```python
from build123d import *

# Parameters (mm, degrees)
F1_DEPTH = 15.748
F2_W     = 38.1
F2_H     = 11.4949838928
F3_DEPTH = 38.1
F4_R     = 19.04999
F6_D     = 15.875
F7_R     = 15.875
F7_R_2   = 7.9375
F8_DEPTH = 3.048


# Not quite as in the source:
# - a fillet or chamfer is up to 0.001 mm smaller than in the source, because OpenCascade refuses the exact size


with BuildPart() as f1:
    # F0 (on Top) → F1 (new body)
    with BuildSketch(Plane.XY):
        with BuildLine():
            Line((-30.7737162879, 0), (58.1262837121, 0))
            ThreePointArc((58.1262837121, 0), (67.1065398331, 3.7197438789), (70.8262837121, 12.7))
            Line((70.8262837121, 12.7), (70.8262837121, 20.574))
            Line((70.8262837121, 20.574), (58.1262837121, 20.574))
            ThreePointArc((58.1262837121, 20.574), (53.3002837121, 25.4), (58.1262837121, 30.226))
            Line((58.1262837121, 30.226), (70.8262837121, 30.226))
            Line((70.8262837121, 30.226), (70.8262837121, 38.1))
            ThreePointArc((70.8262837121, 38.1), (67.1065398331, 47.0802561211), (58.1262837121, 50.8))
            Line((58.1262837121, 50.8), (-30.7737162879, 50.8))
            ThreePointArc((-30.7737162879, 50.8), (-39.753972409, 47.0802561211), (-43.4737162879, 38.1))
            Line((-43.4737162879, 38.1), (-43.4737162879, 30.226))
            Line((-43.4737162879, 30.226), (-30.7737162879, 30.226))
            ThreePointArc((-30.7737162879, 30.226), (-25.9477162879, 25.4), (-30.7737162879, 20.574))
            Line((-30.7737162879, 20.574), (-43.4737162879, 20.574))
            Line((-43.4737162879, 20.574), (-43.4737162879, 12.7))
            ThreePointArc((-43.4737162879, 12.7), (-39.753972409, 3.7197438789), (-30.7737162879, 0))
        make_face()
    extrude(amount=F1_DEPTH)

    # F2 (on face) → F3 (join)
    with BuildSketch(Plane.XY.offset(15.748)):
        with Locations((13.6762837121, 5.7474919464)):
            Rectangle(F2_W, F2_H)
    extrude(amount=F3_DEPTH)

    # F4 (radius 19.05 in the source; OpenCascade refuses exactly that, so slightly less here)
    f4_edges = [f1.edges().sort_by_distance(p)[0] for p in [
        (-5.373716, 5.747492, 53.848),
        (32.726284, 5.747492, 53.848),
    ]]
    fillet(f4_edges, radius=F4_R)

    # F6 (through all)
    with Locations(Plane.XZ):
        with Locations((13.6762837121, 34.798)):
            Hole(F6_D / 2)

    # F7 (on face) → F8 (cut)
    with BuildSketch(Plane.XZ):
        with Locations((13.6762837121, 34.798)):
            Circle(F7_R)
        with Locations((13.6762837121, 34.798)):
            Circle(F7_R_2, mode=Mode.SUBTRACT)
    extrude(amount=-F8_DEPTH, mode=Mode.SUBTRACT)


solid = f1.part
```
Build history of the part. All positions in model axes, mm. A direction names the side the tool comes from. Coordinates: 2 decimals unless noted, no trailing zeros. Write each loop counter-clockwise with the first axis right and the second up, starting at its lowest first coordinate (ties: lowest second). Pieces come first, ordered by that corner, then holes.
1. 3-axis set-ups, long thin cutter, end or side, ignore diameter. For faces 1 (the flat face through (13, 11.495, 26)), 2 (the flat face through (32.726, 6, 25)), 3 (the flat face through (65, 20.574, 8)): which of +Z, -Z, +X, -X, +Y, -Y reach the whole face in a straight line?
Answer block:
face 1: +Z, +X, -X, +Y
face 2: +Z, +X, +Y, -Y
face 3: +Z, -Z, +X
2. Band-saw the part on D-D, the plane x = 25. Give the cut face in (y, z), and give its area (3 significant figures).
Answer block:
outline: (0, 0) - (50.8, 0) - (50.8, 15.75) - (11.49, 15.75) - (11.49, 50.12) - (0, 50.12) - (0, 45.92) - (3.05, 45.92) - (3.05, 23.67) - (0, 23.67) - close
area: 1,130 mm2
3. Drop flat-ended pins along their axis: pin 1 (6.5 mm diameter, centred on x = -34.5, z = 8.5, fed in from +Y); pin 2 (2 mm diameter, centred on x = -26.5, y = 40, fed in from +Z); pin 3 (6.5 mm diameter, centred on x = -38, z = 10.5, fed in from -Y). Give the stop position or say it passes through.
Answer block:
pin 1: stops at y = 50.79
pin 2: stops at z = 15.75
pin 3: stops at y = 0.64
4. Pull direction Y, two halves, no side cores. Call faces 4 (the cylindrical face through (67.205, 46.981, 7.764)), 5 (the cylindrical face through (53.3, 25.3, 7.8)), 6 (the flat face through (13, 26, 0)), 7 (the flat face through (-37, 30.226, 8)): released by +Y, released by -Y, zero draft, split by the parting line, or undercut.
Answer block:
face 4: released by +Y
face 5: undercut
face 6: zero draft
face 7: undercut
5. Band-saw the part on B-B, the plane x = 12. Give the cut face in (y, z).
Answer block:
outline: (0, 0) - (50.8, 0) - (50.8, 15.75) - (11.49, 15.75) - (11.49, 27.04) - (3.05, 27.04) - (3.05, 19.01) - (0, 19.01) - close; (0, 50.58) - (3.05, 50.58) - (3.05, 42.56) - (11.49, 42.56) - (11.49, 53.77) - (0, 53.77) - close
6. Band-saw the part on C-C, the plane z = 47. Give the cut face in (x, y), and give its area (3 significant figures).
Answer block:
outline: (-0.95, 0) - (3.52, 0) - (3.52, 3.05) - (23.83, 3.05) - (23.83, 0) - (28.31, 0) - (28.31, 11.49) - (-0.95, 11.49) - close
area: 274 mm2
7. Band-saw the part on A-A, the plane z = 30.5. Give the cut face in (x, y), and give its area (3 significant figures).
Answer block:
outline: (-5.37, 0) - (-1.61, 0) - (-1.61, 3.05) - (7, 3.05) - (7, 11.49) - (-5.37, 11.49) - close; (20.35, 3.05) - (28.96, 3.05) - (28.96, 0) - (32.73, 0) - (32.73, 11.49) - (20.35, 11.49) - close
area: 232 mm2
8. Drill centre lines: probe 1 along Y at (x, z) = (9, 16.5); probe 2 along X at (y, z) = (6, 16.5); probe 3 along X at (y, z) = (25, 14.5). Where is each one in solid material? Low to high.
Answer block:
probe 1: y = 0 to 11.49
probe 2: x = -5.37 to 32.73
probe 3: x = -25.96 to 53.32
